Part print with two shaded views. Sizes in mm from the minimum x, y, z corner. Round coordinates to 2 decimals unless told otherwise and drop trailing zeros. Write each loop counter-clockwise with the first axis right and the second up, starting at its lowest first coordinate (ties: lowest second). Pieces come first, ordered by that corner, then holes. Notation, with made-up numbers: (-28.5, 12) -> (17.5, 12) arc R20 cw to (17.5, 37) -> close; hole circle Ø1 at (65, -17.5). An arc over 180 degrees is marked (long way). Return JSON: item names as keys, results as strings.
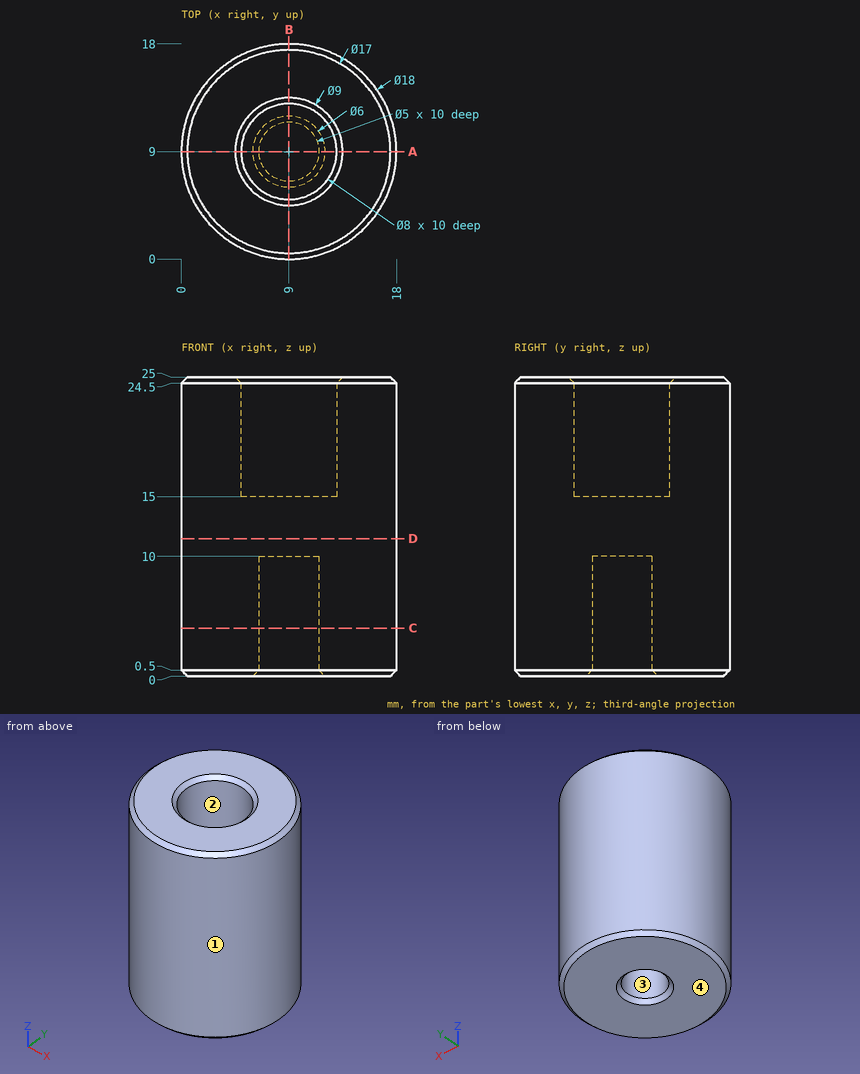
Q1. Saw through at C-C on z = 4. List the corners of the cut face in (x, y), then the cut area to 3 significant figures.
Verdict:
{"outline": "circle Ø18 at (9, 9); hole circle Ø5 at (9, 9)", "area": "235 mm²"}
Q2. Wall check: L1, parallel to Y at x = 9, z = 7.75; L2, parallel to Y at x = 9, z = 18.75; L3, parallel to Z at x = 6, y = 8.25. Give the ranges that are in metal, low to high.
Verdict:
{"L1": "y = 0 to 6.5, 11.5 to 18", "L2": "y = 0 to 5, 13 to 18", "L3": "z = 0 to 15"}
Q3. Two-plate mould, pull along X, no slides. Class the marked faces 1, 2, 3 and 4: +X half, -X half, draft (parallel to the pull), parting line (faces both ways), or undercut.
Verdict:
{"face 1": "parting line", "face 2": "undercut", "face 3": "undercut", "face 4": "draft"}
Q4. Saw through at A-A on y = 9. List the corners of the cut face in (x, z), then the cut area to 3 significant figures.
Verdict:
{"outline": "(0, 0.5) -> (0.5, 0) -> (6, 0) -> (6.5, 0.5) -> (6.5, 10) -> (11.5, 10) -> (11.5, 0.5) -> (12, 0) -> (17.5, 0) -> (18, 0.5) -> (18, 24.5) -> (17.5, 25) -> (13.5, 25) -> (13, 24.5) -> (13, 15) -> (5, 15) -> (5, 24.5) -> (4.5, 25) -> (0.5, 25) -> (0, 24.5) -> close", "area": "319 mm²"}
Q5. Saw through at D-D on z = 11.5. List the corners of the cut face in (x, y), then the cut area to 3 significant figures.
Verdict:
{"outline": "circle Ø18 at (9, 9)", "area": "254 mm²"}
Q6. Pin check, flat tips, straight feed: pin 1 Ø4 at (y, z) = (4.5, 10.5) entering from +X; pin 2 Ø3 at (x, y) = (9, 9) entering from -Z; pin 3 Ø5 at (y, z) = (15, 13.5) entering from +X. Stop position of each tip, or through.
Verdict:
{"pin 1": "stops at x = 17.65", "pin 2": "stops at z = 10", "pin 3": "stops at x = 17.29"}
